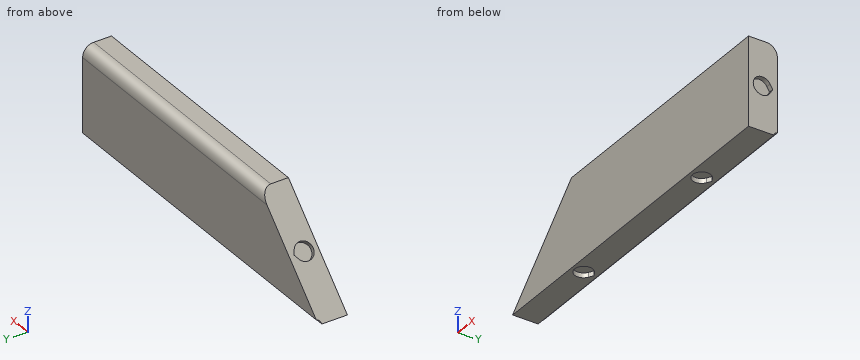
from build123d import *

# Parameters (mm, degrees)
EXTRUDE_1_DEPTH     = 13
SWEEP_START         = -80
SWEEP_1_DEPTH       = 160
SKETCH_6_R          = 4.075
CUT_EXTRUDE_1_DEPTH = 2.15
FILLET_1_R          = 5
SKETCH_7_R          = 4.075
CUT_EXTRUDE_2_DEPTH = 2.15
SKETCH_8_R          = 4.075
CUT_EXTRUDE_3_DEPTH = 2.15


# Read off the part's stored shape, not the designer's step: Вырез-По траектории1
with BuildPart() as part:
    # Эскиз1 → Бобышка-Вытянуть1 (new body)
    with BuildSketch(Plane(origin=(0, 0, 0), x_dir=(1, 0, 0), z_dir=(0, 1, 0))):
        Polygon((-40, -20), (80, -20), (80, 20), (-80, 20), align=None)
    extrude(amount=-EXTRUDE_1_DEPTH)

    # Вырез-По траектории1 outline → Вырез-По траектории1 (cut)
    with BuildSketch(Plane.YZ.offset(SWEEP_START)):
        with BuildLine():
            ThreePointArc((0, -18.5), (-1.060660172, -18.939339828), (-1.5, -20))
            Line((-1.5, -20), (0, -20))
            Line((0, -20), (0, -18.5))
        make_face()
    extrude(amount=SWEEP_1_DEPTH, mode=Mode.SUBTRACT)

    # Эскиз6 → Вырез-Вытянуть1 (cut)
    with BuildSketch(Plane(origin=(0, 0, -20), x_dir=(-1, 0, 0), z_dir=(0, 0, -1))):
        with Locations((-40, -7.565202347)):
            Circle(SKETCH_6_R)
        with BuildLine():
            Line((-40, -2.859797653), (-42.0375, -4.036148827))
            ThreePointArc((-42.0375, -4.036148827), (-40, -3.490202347), (-37.9625, -4.036148827))
            Line((-37.9625, -4.036148827), (-40, -2.859797653))
        make_face()
        with Locations((40, -7.565202347)):
            Circle(SKETCH_6_R)
        with BuildLine():
            ThreePointArc((37.9625, -4.036148827), (40, -3.490202347), (42.0375, -4.036148827))
            Line((42.0375, -4.036148827), (40, -2.859797653))
            Line((40, -2.859797653), (37.9625, -4.036148827))
        make_face()
    extrude(amount=-CUT_EXTRUDE_1_DEPTH, mode=Mode.SUBTRACT)

    # Скругление1
    fillet_1_edges = [part.edges().sort_by_distance(p)[0] for p in [
        (20, 0, 20),
    ]]
    fillet(fillet_1_edges, radius=FILLET_1_R)

    # Эскиз7 → Вырез-Вытянуть2 (cut)
    with BuildSketch(Plane.ZY.offset(-80)):
        with Locations((0, -6.815202347)):
            Circle(SKETCH_7_R)
        with BuildLine():
            Line((2.0375, -3.286148827), (0, -2.109797653))
            Line((0, -2.109797653), (-2.0375, -3.286148827))
            ThreePointArc((-2.0375, -3.286148827), (0, -2.740202347), (2.0375, -3.286148827))
        make_face()
    extrude(amount=CUT_EXTRUDE_2_DEPTH, mode=Mode.SUBTRACT)

    # Эскиз8 → Вырез-Вытянуть3 (cut)
    with BuildSketch(Plane(origin=(-30, 0, 30), x_dir=(0.7071067811865515, 0, 0.7071067811865436), z_dir=(-0.7071067811865436, 0, 0.7071067811865515))):
        with Locations((-42.426406871, -6.815202347)):
            Circle(SKETCH_8_R)
        with BuildLine():
            Line((-42.426406871, -2.109797653), (-44.463906871, -3.286148827))
            ThreePointArc((-44.463906871, -3.286148827), (-42.426406871, -2.740202347), (-40.388906871, -3.286148827))
            Line((-40.388906871, -3.286148827), (-42.426406871, -2.109797653))
        make_face()
    extrude(amount=-CUT_EXTRUDE_3_DEPTH, mode=Mode.SUBTRACT)


solid = part.part
Work out the finished part from the listing and answer in its coordinate system (mm). Coordinates: 2 decimals unless noted, no trailing zeros. Write each loop counter-clockwise with the first axis right and the second up, starting at its lowest first coordinate (ties: lowest second). Pieces come first, ordered by that corner, then holes.
1. Flat-ended cylindrical pins translate along their axes: pin 1 (2.5 mm diameter, centred on y = -5, z = -1.5, fed in from +X); pin 2 (7.5 mm diameter, centred on x = 40, y = -7.57, fed in from -Z); pin 3 (2 mm diameter, centred on y = -5, z = 15, fed in from -X). Find the tip coordinate at first contact, or state that the pin passes through.
Results list:
pin 1: stops at x = 77.85
pin 2: stops at z = -17.85
pin 3: stops at x = -46
2. Consider line 1 along X through (y, z) = (-10.25, -18); line 2 along Z through (x, y) = (31, -4.5); line 3 along Y through (x, z) = (-40, -19.45). Determine where each line is inside the solid, lowest interval first.
Results list:
line 1: x = -78 to -43.07, -36.93 to 36.93, 43.07 to 80
line 2: z = -20 to 19.97
line 3: y = -13 to -11.64, -2.86 to -1.4
3. The part is cut by section D-D, the plane z = 6.5. Write down the section's boundary in (x, y).
Results list:
outline: (-53.5, -13) - (80, -13) - (80, 0) - (-53.5, 0) - close
4. The part is cut by section B-B, the plane z = -16.5. Write down the section's boundary in (x, y), and give its area (3 significant figures).
Results list:
outline: (-76.5, -13) - (80, -13) - (80, 0) - (-76.5, 0) - close
area: 2,030 mm2
5. The part is cut by section A-A, the plane x = -49. Write down the section's boundary in (y, z).
Results list:
outline: (-13, -20) - (-1.5, -20) arc R1.5 cw to (0, -18.5) - (0, 11) - (-13, 11) - close
6. The part is cut by section C-C, the plane y = -9. Write down the section's boundary in (x, z), and give its area (3 significant figures).
Results list:
outline: (-80, -20) - (-43.81, -20) - (-43.81, -17.85) - (-36.19, -17.85) - (-36.19, -20) - (36.19, -20) - (36.19, -17.85) - (43.81, -17.85) - (43.81, -20) - (80, -20) - (80, -3.44) - (77.85, -3.44) - (77.85, 3.44) - (80, 3.44) - (80, 20) - (-40, 20) - (-57.57, 2.43) - (-56.05, 0.91) - (-60.91, -3.95) - (-62.43, -2.43) - close
area: 5,540 mm2
